Autodesk Inventor part; units mm, degrees
ref_plane "YZ Plane" through (0, 0, 0) normal (1, 0, 0) x (0, 1, 0)
ref_plane "XZ Plane" through (0, 0, 0) normal (0, 1, 0) x (-1, 0, 0)
ref_plane "XY Plane" through (0, 0, 0) normal (0, 0, 1) x (1, 0, 0)
sketch "Sketch1" plane through (0, 0, 0) normal (1, 0, 0) x (0, 1, 0)
  circle A0 centre (-4, -4) radius 2
  circle A1 centre (78.5, 78.5) radius 85
  circle A2 centre (161, -4) radius 2
  circle A3 centre (-4, 161) radius 2
  circle A4 centre (161, 161) radius 2
  line L0 (157, 170) -> (0, 170)
  arc A5 (0, 170) -> (-13, 157) centre (0, 157) ccw
  line L1 (-13, 157) -> (-13, 0)
  arc A6 (-13, 0) -> (0, -13) centre (0, 0) ccw
  line L2 (0, -13) -> (157, -13)
  arc A7 (157, -13) -> (170, 0) centre (157, 0) ccw
  line L3 (170, 0) -> (170, 157)
  arc A8 (170, 157) -> (157, 170) centre (157, 157) ccw
  line L4 (-4, 161) -> (161, 161) construction
  line L5 (161, 161) -> (161, -4) construction
  line L6 (161, -4) -> (-4, -4) construction
  line L7 (-4, -4) -> (-4, 161) construction
  line L8 (-4, 161) -> (161, -4) construction
  line L9 (-13, 78.5) -> (78.5, 78.5) construction
  line L10 (78.5, 78.5) -> (170, 78.5) construction
  dimension "d10" = 183
  dimension "d11" = 183
  dimension "d12" = 165
  dimension "d13" = 165
  dimension "d15" = 13
  dimension "d16" = 4
  dimension "d17" = 170
extrude "Extrusion1" add sketch "Sketch1" along normal blind 2.75
sketch "Sketch2" plane through (2.75, 0, 0) normal (1, 0, 0) x (0, 0, -1)
  line L0 (0, 170) -> (-157, 170)
  line L1 (-146.1, 170) -> (-131.1, 170)
  line L2 (-131.1, 170) -> (-131.1, 166.5)
  line L3 (-131.1, 166.5) -> (-146.1, 166.5)
  line L4 (-146.1, 166.5) -> (-146.1, 170)
  line L5 (-116.1, 170) -> (-101.1, 170)
  line L6 (-101.1, 170) -> (-101.1, 166.5)
  line L7 (-101.1, 166.5) -> (-116.1, 166.5)
  line L8 (-116.1, 166.5) -> (-116.1, 170)
  line L9 (-47.1, 170) -> (-32.1, 170)
  line L10 (-32.1, 170) -> (-32.1, 166.5)
  line L11 (-32.1, 166.5) -> (-47.1, 166.5)
  line L12 (-47.1, 166.5) -> (-47.1, 170)
  line L13 (-2.1, 170) -> (-17.1, 170)
  line L14 (-17.1, 170) -> (-17.1, 166.5)
  line L15 (-17.1, 166.5) -> (-2.1, 166.5)
  line L16 (-2.1, 166.5) -> (-2.1, 170)
  circle A0 centre (-161, 161) radius 2
  point P0 (0, 0)
  dimension "d2" = 15
  dimension "d3" = 30
  dimension "d4" = 69
  dimension "d5" = 30
  dimension "d6" = 3.5
  dimension "d7" = 14.9
extrude "Extrusion2" cut sketch "Sketch2" against normal blind 10 contours L16 L15 L14 L0 | L2 L3 L4 L0 | L6 L7 L8 L0 | L10 L11 L12 L0
sketch "Sketch3" plane through (2.75, 0, 0) normal (1, 0, 0) x (0, 0, -1)
  line L0 (-56.4, -11.425) -> (-41.4, -11.425)
  line L1 (-41.4, -11.425) -> (-41.4, -8.675)
  line L2 (-41.4, -8.675) -> (-56.4, -8.675)
  line L3 (-56.4, -8.675) -> (-56.4, -11.425)
  line L4 (-26.4, -11.425) -> (-11.4, -11.425)
  line L5 (-11.4, -11.425) -> (-11.4, -8.675)
  line L6 (-11.4, -8.675) -> (-26.4, -8.675)
  line L7 (-26.4, -8.675) -> (-26.4, -11.425)
  line L8 (-106.4, -11.425) -> (-121.4, -11.425)
  line L9 (-121.4, -11.425) -> (-121.4, -8.675)
  line L10 (-121.4, -8.675) -> (-106.4, -8.675)
  line L11 (-106.4, -8.675) -> (-106.4, -11.425)
  line L12 (-136.4, -11.425) -> (-151.4, -11.425)
  line L13 (-151.4, -11.425) -> (-151.4, -8.675)
  line L14 (-151.4, -8.675) -> (-136.4, -8.675)
  line L15 (-136.4, -8.675) -> (-136.4, -11.425)
  line L16 (-157, -13) -> (0, -13)
  circle A0 centre (-161, -4) radius 2
  point P0 (0, 0)
  dimension "d18" = 1.575
  dimension "d19" = 30
  dimension "d20" = 65
  dimension "d21" = 30
  dimension "d22" = 2.75
  dimension "d23" = 9.6
  dimension "d26" = 15
extrude "Extrusion3" cut sketch "Sketch3" against normal blind 10 contours L3 L2 L1 L0 | L7 L6 L5 L4 | L8 L9 L10 L11 | L12 L13 L14 L15
sketch "Sketch4" plane through (2.75, 0, 0) normal (1, 0, 0) x (0, 0, -1)
  line L0 (-75.85, 147) -> (-73.1, 147)
  line L1 (-73.1, 147) -> (-73.1, 162)
  line L2 (-73.1, 162) -> (-75.85, 162)
  line L3 (-75.85, 162) -> (-75.85, 147)
  line L4 (-78.85, 144) -> (-70.1, 144)
  line L5 (-70.1, 144) -> (-63.1, 165)
  line L6 (-63.1, 165) -> (-85.85, 165)
  line L7 (-85.85, 165) -> (-78.85, 144)
  line L8 (-47.1, 170) -> (-101.1, 170)
  line L9 (-47.1, 166.5) -> (-47.1, 170)
  point P0 (0, 0)
  dimension "d27" = 8
  dimension "d28" = 26
  dimension "d29" = 2.75
  dimension "d30" = 15
  dimension "d31" = 3
  dimension "d32" = 3
  dimension "d33" = 3
  dimension "d34" = 10
  dimension "d35" = 10
  dimension "d36" = 5
extrude "Extrusion4" add sketch "Sketch4" against normal up to surface (2.75 mm away)
fillet "Fillet1" radius 2 4 edges at (1.375, 144, 78.85) (1.375, 144, 70.1) (1.375, 163.2307, 85.2602) (1.375, 162.2566, 64.0145)
sketch "Sketch5" plane through (2.75, 0, 0) normal (1, 0, 0) x (0, 0, -1)
  circle A0 centre (-11, 153) radius 7.5
  circle A1 centre (4, 161) radius 2
  point P0 (0, 0)
  dimension "d40" = 15
  dimension "d41" = 15
  dimension "d42" = 8
extrude "Extrusion5" cut sketch "Sketch5" against normal blind 10 contours A0
properties part number "TrayPanelD_180mm"
The listing builds one solid part. Answer for the finished solid, in the listing's coordinates (mm). A direction names the side the tool comes from. Give positions to 0.01 mm unless a question says otherwise; leave off trailing zeros. Write each loop counter-clockwise with the first axis right and the second up, starting at its lowest first coordinate (ties: lowest second). Pieces come first, ordered by that corner, then holes. Notation, with made-up numbers: (83.5, 48.25) -> (129.5, 48.25) arc R11 cw to (129.5, 57.25) -> close; hole circle Ø6 at (36, 53.5). An arc over 180 degrees is marked (long way). Use one line per item in the form item = value.
1) Section B-B on z = 133.5 is taken. Write down the section's boundary in (x, y), plus the area to 3 significant figures.
Result:
outline = (0, -13) -> (2.75, -13) -> (2.75, 13.69) -> (0, 13.69) -> close; (0, 143.31) -> (2.75, 143.31) -> (2.75, 166.5) -> (0, 166.5) -> close
area = 137 mm²
2) A tool of negligible diameter and unlimited length cuts with its end or side. For faces 4 (the cylindrical face through (1.356, 166.293, -9.091)), 5 (the flat face through (1.39, 153.66, 82.07)), from which of +Z, -Z, +X, -X, +Y, -Y can it reach the whole face along a straight path? Write none if from no direction.
Result:
face_4 = -Z, +X, -X, +Y
face_5 = +X, -X
3) For a pull along Y with two mould halves and no side action, classify faces 1 (the cylindrical face through (1.4, -6.5, 78.9)), 2 (the flat face through (2.75, 153, 79)), 3 (the cylindrical face through (1.356, -9.293, 166.091)) as +Y half, -Y half, draft (parallel to the pull), parting line (faces both ways), or undercut.
Result:
face_1 = undercut
face_2 = draft
face_3 = -Y half
4) Section C-C on y = 153 is taken. Write down the section's boundary in (x, z), plus the area to 3 significant figures.
Result:
outline = (0, -13) -> (2.75, -13) -> (2.75, 3.5) -> (0, 3.5) -> close; (0, 18.5) -> (2.75, 18.5) -> (2.75, 37.58) -> (0, 37.58) -> close; (0, 67.1) -> (2.75, 67.1) -> (2.75, 73.1) -> (0, 73.1) -> close; (0, 75.85) -> (2.75, 75.85) -> (2.75, 81.85) -> (0, 81.85) -> close; (0, 119.42) -> (2.75, 119.42) -> (2.75, 170) -> (0, 170) -> close
area = 270 mm²
5) Straight lines are drawn through the part: probe 1 along Y at (x, z) = (1.65, 46) (3 decimals); probe 2 along Y at (x, z) = (1.9, 25) (3 decimals); probe 3 along Z at (x, y) = (1.9, 78.5). For each, find the intervals that lie inside material, in ascending order.
Result:
probe_1 = -13 to -11.425, -8.675 to -0.041, 157.041 to 166.5
probe_2 = -13 to -11.425, -8.675 to 12.449, 144.551 to 170
probe_3 = -13 to -6.5, 163.5 to 170
6) Section D-D on z = 49.5 is taken. Write down the section's boundary in (x, y) (3 decimals), plus the area to 3 significant figures.
Result:
outline = (0, -13) -> (2.75, -13) -> (2.75, -11.425) -> (0, -11.425) -> close; (0, -8.675) -> (2.75, -8.675) -> (2.75, -1.4) -> (0, -1.4) -> close; (0, 158.4) -> (2.75, 158.4) -> (2.75, 170) -> (0, 170) -> close
area = 56.2 mm²
7) Section A-A on y = 42.5 is taken. Write down the section's boundary in (x, z).
Result:
outline = (0, -13) -> (2.75, -13) -> (2.75, 1.5) -> (0, 1.5) -> close; (0, 155.5) -> (2.75, 155.5) -> (2.75, 170) -> (0, 170) -> close
8) Each of these flat-tipped pins is pushed along its axis until it touches: P1, Ø1.4, axis at x = 2, y = -9.5, coming from the +Z side; P2, Ø6.5, axis at y = 161, z = -4, coming from the +X side; P3, Ø1.4, axis at x = 0.5, y = -9.5, coming from the -Z side; P4, Ø0.8, axis at x = 0.5, z = 41.5, coming from the +Y side. Where does it stop, or does it pass through?
Result:
P1 = 166.57
P2 = 2.75
P3 = -9.57
P4 = 166.5
